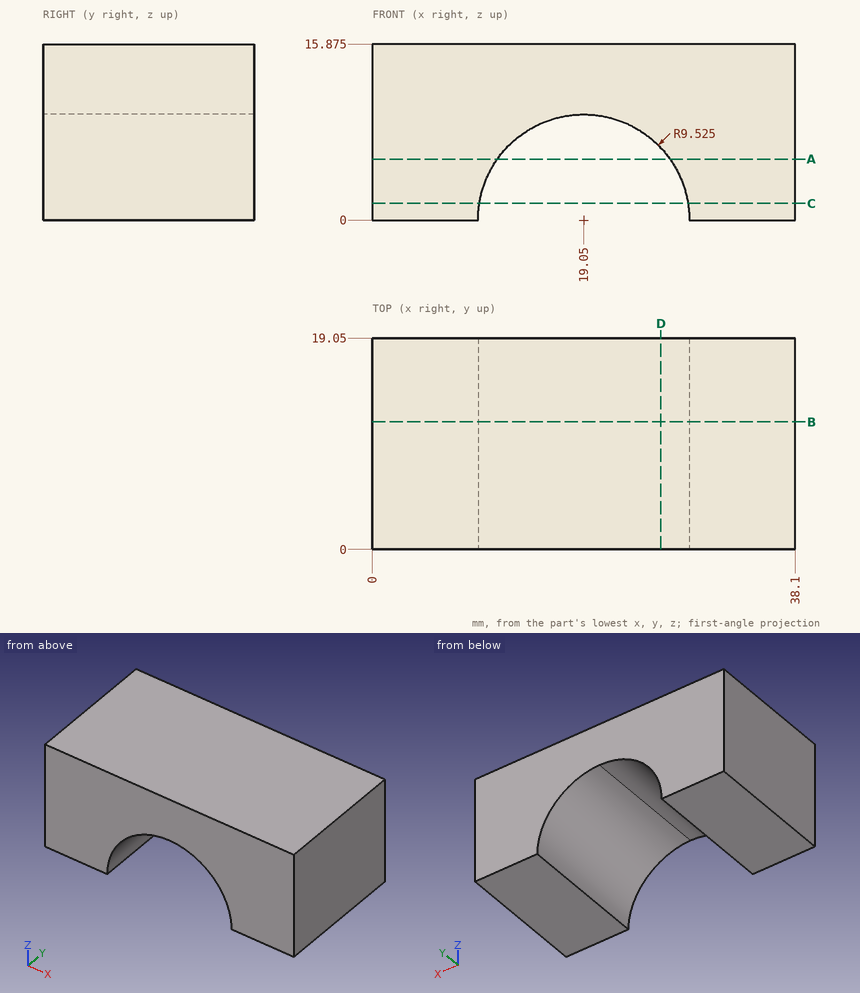
Can you work these out from the drawing? Everything is in mm from the part's minimum corner. Coordinates: 2 decimals unless noted, no trailing zeros. Order: outer loops, then holes, each group sorted by start corner. A loop starts at its lowest first (then second) coordinate and runs counter-clockwise, first axis right, second up. Notation, with made-up numbers: (21.25, -12) -> (70.25, -12) arc R28 cw to (70.25, 9) -> close; hole circle Ø2 at (64.5, -30). An arc over 180 degrees is marked (long way). Use one line per item in the form item = value.
Q1. Imagine slicing it at C-C, the plane z = 1.5. List the corners of the cut face in (x, y) for me.
From the geometry:
outline = (0, 0) -> (9.64, 0) -> (9.64, 19.05) -> (0, 19.05) -> close; (28.46, 0) -> (38.1, 0) -> (38.1, 19.05) -> (28.46, 19.05) -> close
Q2. Will these pins go through, and if not, where does the flat tip stop? P1, Ø2, axis at y = 7, z = 9.5, coming from the -X side; P2, Ø2, axis at x = 22.5, y = 3.5, coming from the -Z side; P3, Ø2, axis at x = 26.5, y = 7.5, coming from the -Z side.
From the geometry:
P1 = 0
P2 = 8.42
P3 = 4.4
Q3. I need wall thicknesses on L1, parallel to X at y = 14.75, z = 5; L2, parallel to X at y = 2, z = 8.75; L3, parallel to Z at x = 19, y = 1 (3 decimals). Which ranges of each line are inside material? Lowest first, please.
From the geometry:
L1 = 0 to 10.94, 27.16 to 38.1
L2 = 0 to 15.29, 22.81 to 38.1
L3 = 9.525 to 15.875
Q4. Imagine slicing it at B-B, the plane y = 11.5. List the corners of the cut face in (x, z) for me (3 decimals).
From the geometry:
outline = (0, 0) -> (9.525, 0) arc R9.525 cw to (28.575, 0) -> (38.1, 0) -> (38.1, 15.875) -> (0, 15.875) -> close
Q5. Imagine slicing it at A-A, the plane z = 5.5. List the corners of the cut face in (x, y) for me.
From the geometry:
outline = (0, 0) -> (11.27, 0) -> (11.27, 19.05) -> (0, 19.05) -> close; (26.83, 0) -> (38.1, 0) -> (38.1, 19.05) -> (26.83, 19.05) -> close
Q6. Imagine slicing it at D-D, the plane x = 26. List the corners of the cut face in (y, z) for me (3 decimals), then the cut area to 3 significant figures.
From the geometry:
outline = (0, 6.513) -> (19.05, 6.513) -> (19.05, 15.875) -> (0, 15.875) -> close
area = 178 mm²
